Work out the finished part from the listing and answer in its coordinate system (mm). Face numbers are marked on the shaded views. A direction names the side the tool comes from. Round coordinates to 2 decimals unless told otherwise and drop trailing zeros. Order: outer loops, then holes, each group sorted by start corner. A loop starts at its lowest first (then second) coordinate and runs counter-clockwise, first axis right, second up. Notation, with made-up numbers: (31.5, 82.25) -> (83.5, 82.25) arc R17 cw to (83.5, 114.25) -> close; hole circle Ø2 at (29.25, 78). An arc over 180 degrees is marked (long way). Use a Markdown table: item, result. Add a question column.
Item 1: For a pull along X with two mould halves and no side action, classify the marked faces 1, 2 and 3 as +X half, -X half, draft (parallel to the pull), parting line (faces both ways), or undercut.
Item 2: A cutting plane is placed at A-A, the plane y = -38.5. Determine the outline of the cut face in (x, z), plus the area to 3 significant figures.
Item 3: Flat-ended cylindrical pins translate along their axes: P1, Ø6, axis at x = 28, y = -19.5, coming from the +Z side; P2, Ø1, axis at y = -24.5, z = 60.5, coming from the +X side; P3, Ø4, axis at y = -6.5, z = 30.5, coming from the -X side. Find the tip coordinate at first contact, or state that the pin passes through.
Item 4: Find the intervals of material crossed by L1, parallel to Y at x = 25, z = 27.5; L2, parallel to X at y = -46, z = -5.5; L3, parallel to Z at x = 9, y = -43.5, in increasing order. Write a range as [from, to].
Item 5: A tool of negligible diameter and unlimited length cuts with its end or side. For the marked faces 4, 5 and 6, from which of +Z, -Z, +X, -X, +Y, -Y can it reach the whole face along a straight path? Write none if from no direction.
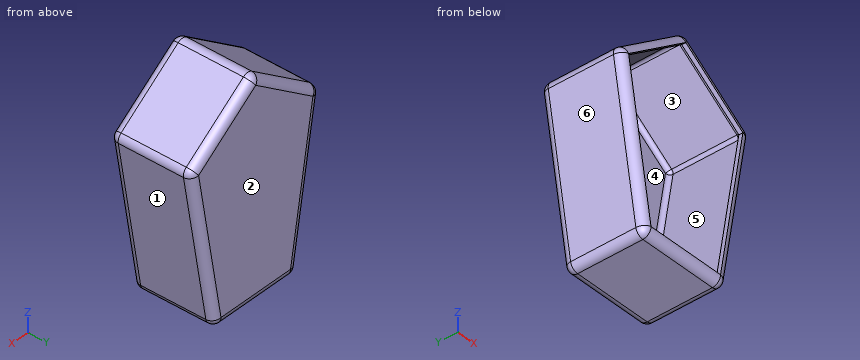
from build123d import *

# Parameters (mm, degrees)
F1_DEPTH = 50.8
F2_R     = 5.08
F3_T     = -2.54


# Not quite as in the source:
# - a shell that OpenCascade refuses in one call is made with other operations: the cavity is built on its own and cut out


with BuildPart() as f1:
    # F0 (on Front) → F1 (new body)
    with BuildSketch(Plane.XZ):
        Polygon((-46.4516356587, 59.1254718602), (-29.1618652595, -40.9925776591), (-21.6381347405, -40.9925776591), (21.6381347405, -40.9925776591), (29.1618652595, -40.9925776591), (46.4516356587, 59.1254718602), (0, 92.9853990674), align=None)
    extrude(amount=F1_DEPTH)

    # F2
    f2_edges = [f1.edges().sort_by_distance(p)[0] for p in [
        (23.225818, -50.8, 76.055435),
        (-23.225818, -50.8, 76.055435),
        (-37.80675, -50.8, 9.066447),
        (0, -50.8, -40.992578),
        (37.80675, -50.8, 9.066447),
        (29.161865, -25.4, -40.992578),
        (46.451636, -25.4, 59.125472),
        (37.80675, 0, 9.066447),
        (23.225818, 0, 76.055435),
        (-23.225818, 0, 76.055435),
        (-37.80675, 0, 9.066447),
        (0, 0, -40.992578),
        (-46.451636, -25.4, 59.125472),
        (-29.161865, -25.4, -40.992578),
        (0, -25.4, 92.985399),
    ]]
    fillet(f2_edges, radius=F2_R)

    # F3: a shell. OpenCascade refuses it in one call, so the cavity is built on its own and cut out:
    # the body offset inwards by the wall thickness, plus a prism from it out through each open face.
    f3_core = offset(f1.part, amount=F3_T, mode=Mode.PRIVATE)
    f3_exits = [f3_core.faces().sort_by_distance(p)[0] for p in [
        (0, -48.26, 23.00503),
    ]]
    add(f3_core, mode=Mode.SUBTRACT)
    extrude(f3_exits, amount=-F3_T, mode=Mode.SUBTRACT)


solid = f1.part
Reported:
| question | item | result |
|---|---|---|
| 1 | face 1 | +X half |
| 1 | face 2 | draft |
| 1 | face 3 | undercut |
| 2 | outline | (-45.91, 56.02) -> (-29.89, -36.78) arc R5.08 ccw to (-24.88, -40.99) -> (24.88, -40.99) arc R5.08 ccw to (29.89, -36.78) -> (45.91, 56.02) arc R5.08 ccw to (43.9, 60.98) -> (2.99, 90.8) arc R5.08 ccw to (-2.99, 90.8) -> (-43.9, 60.98) arc R5.08 ccw to start; hole (-43.41, 56.45) -> (-27.39, -36.34) arc R2.54 ccw to (-24.88, -38.45) -> (24.88, -38.45) arc R2.54 ccw to (27.39, -36.34) -> (43.41, 56.45) arc R2.54 ccw to (42.4, 58.93) -> (1.5, 88.75) arc R2.54 ccw to (-1.5, 88.75) -> (-42.4, 58.93) arc R2.54 ccw to start |
| 2 | area | 923 mm² |
| 3 | P1 | z = 74.76 |
| 3 | P2 | x = 44.92 |
| 3 | P3 | x = -41.85 |
| 4 | L1 | [-2.54, 0] |
| 4 | L2 | [-35.28, -32.7], [32.7, 35.28] |
| 4 | L3 | [-40.99, -38.45], [83.28, 86.43] |
| 5 | face 4 | -Y |
| 5 | face 5 | none |
| 5 | face 6 | -Z, -X, +Y, -Y |
